from build123d import *

# Parameters (mm, degrees)
CYLINDER1708_R              = 74
CYLINDER1708_DEPTH          = 40
BOX671_W                    = 42
BOX671_H                    = 62
BOX671_DEPTH                = 50
COMPOUND846_PLACEMENT_ANGLE = 225
BOX672_W                    = 54
BOX672_H                    = 68
BOX672_DEPTH                = 9
COMPOUND847_PLACEMENT_ANGLE = 225
CHAMFER053_SIZE             = 3


with BuildPart() as obj1:
    # Cylinder1708 → Cylinder1708 (new body)
    with BuildSketch(Plane.XY.offset(44)):
        Circle(CYLINDER1708_R)
    extrude(amount=CYLINDER1708_DEPTH)


with BuildPart() as compound846:
    # Box671 → Box671 (new body)
    with BuildSketch(Plane(origin=(-21.001071, 60.005081, 31), x_dir=(1, 0, 0), z_dir=(0, 0, 1))):
        with Locations((21, 31)):
            Rectangle(BOX671_W, BOX671_H)
    extrude(amount=BOX671_DEPTH)


with BuildPart() as compound846_1:
    # Compound846 placement: moved
    add(compound846.part.moved(Location((0, 0, 1))).rotate(Axis((0, 0, 1), (0, 0, 1)), COMPOUND846_PLACEMENT_ANGLE))


with BuildPart() as chamfer053:
    # Box672 → Box672 (new body)
    with BuildSketch(Plane(origin=(-27.004408, 59.99801, 75), x_dir=(1, 0, 0), z_dir=(0, 0, 1))):
        with Locations((27, 34)):
            Rectangle(BOX672_W, BOX672_H)
    extrude(amount=BOX672_DEPTH)


with BuildPart() as chamfer053_1:
    # Compound847 placement: moved
    add(chamfer053.part.rotate(Axis((0, 0, 0), (0, 0, 1)), COMPOUND847_PLACEMENT_ANGLE))

    # Cut489: cut Compound846
    add(compound846_1.part, mode=Mode.SUBTRACT)

    # Cut490: cut obj1
    add(obj1.part, mode=Mode.SUBTRACT)

    # Chamfer053
    chamfer053_edges = [chamfer053_1.edges().sort_by_distance(p)[0] for p in [
        (109.603261, -71.413261, 79.5),
        (71.419495, -109.597027, 79.5),
    ]]
    chamfer(chamfer053_edges, length=CHAMFER053_SIZE)


solid = chamfer053_1.part
Geometry: final body of the model. Coordinates: model frame, mm. A direction names the side the tool comes from. Round coordinates to 2 decimals unless told otherwise and drop trailing zeros. Loops run counter-clockwise (first coordinate to the right, second up) from the corner with the lowest first, then second, coordinate; pieces in that order, holes last. Notation, with made-up numbers: M -40,-7 L 0,-7 A28 cw 0,29 Z; hole C 71,-30.5 d1. An arc over 180 degrees is marked long. Put each result on its own line as item: value. Start each with the question number.
(1) Draft query along X for faces 3 (the face through (49.187, -87.364, 79.437)), 4 (the face through (71, -107.476, 79)), 5 (the face through (107.482, -71, 79)), 6 (the face through (69, -68, 82)). Return one class per face: +X half, -X half, draft (parallel to the pull), parting line (faces both ways), or undercut.
(2) Section query A-A (z = 76). Return loops of the section in (x, y), then the cut area to 3 significant figures.
(3) Set-up query: faces 1 (the face through (86.48, -86.06, 78.45)), 2 (the face through (90.749, -90.268, 79.437)). Return all of +Z, -Z, +X, -X, +Y, -Y with unobstructed straight access to the full face (end or side cutting, diameter ignored); none if empty.
(4) Section query B-B (x = 74.5). Return loops of the section in (y, z).
(5) Material intervals for line 1 along Z through (x, y) = (60, -45.5); line 2 along X through (y, z) = (-67, 81.5); line 3 along Y through (x, z) = (82, 77), sorted ascending. Write a range as [from, to].
(6) Section query C-C (y = -89.5). Return loops of the section in (x, z), then the cut area to 3 significant figures.
(7) Contact query for flat-ended pins moving along their axis: pin 1 Ø4 at (x, y) = (78, -58.5) entering from -Z; pin 2 Ø1.5 at (y, z) = (-45, 78) entering from +X; pin 3 Ø2 at (y, z) = (-76.5, 79.5) entering from -X. Output: stop coordinate, or through.
(8) Section query D-D (x = 49.5). Return loops of the section in (y, z), then the cut area to 3 significant figures.
Findings below:
1. face 3: -X half
1. face 4: draft
1. face 5: +X half
1. face 6: undercut
2. outline: M 29.63,-67.81 L 69.3,-107.48 L 73.54,-107.48 L 107.48,-73.53 L 107.48,-69.29 L 67.81,-29.62 A74 cw 65.02,-35.32 L 101.12,-71.42 L 71.42,-101.12 L 35.33,-65.02 A74 cw Z
2. area: 939 mm2
3. face 1: -Z
3. face 2: +Z, -Z, +X, -Y
4. outline: M -106.52,75 L -98.04,75 L -98.04,82 L -44.8,82 L -44.8,75 L -36.31,75 L -36.31,84 L -106.52,84 Z
5. line 1: z = [82, 84]
5. line 2: x = [31.42, 37.3], [96.7, 105.19]
5. line 3: y = [-99.02, -90.54], [-52.3, -43.81]
6. outline: M 51.32,75 L 59.8,75 L 59.8,82 L 83.04,82 L 83.04,75 L 91.52,75 L 91.52,84 L 51.32,84 Z
6. area: 199 mm2
7. pin 1: stops at z = 82
7. pin 2: stops at x = 83.94
7. pin 3: stops at x = 37.32
8. outline: M -87.68,75 L -79.2,75 L -79.2,82 L -55.01,82 L -55.01,84 L -87.68,84 Z
8. area: 125 mm2
